from build123d import *

# Parameters (mm, degrees)
EXTRUDE_1_DEPTH = 46
SKETCH_2_R      = 5
EXTRUDE_2_DEPTH = 113
FILLET_1_R      = 3


with BuildPart() as part:
    # 草圖1 → 填料-伸長1 (new body)
    with BuildSketch(Plane.XY):
        Polygon((-15, 1.25), (-13.544119063, 5.25), (13.544119063, 5.25), (15, 1.25), (15, -1.25), (13.544119063, -5.25), (-13.544119063, -5.25), (-15, -1.25), align=None)
    extrude(amount=EXTRUDE_1_DEPTH)

    # 草圖2 → 填料-伸長2 (add)
    with BuildSketch(Plane(origin=(0, 0, 0), x_dir=(-1, 0, 0), z_dir=(0, 0, -1))):
        with Locations((7, 0)):
            Circle(SKETCH_2_R)
    extrude(amount=EXTRUDE_2_DEPTH)

    # 圓角1
    fillet_1_edges = [part.edges().sort_by_distance(p)[0] for p in [
        (-2, 0, -113),
    ]]
    fillet(fillet_1_edges, radius=FILLET_1_R)


solid = part.part
Verification items for the finished model (mm, model axes). A direction names the side the tool comes from. Coordinates: 2 decimals unless noted, no trailing zeros. Loops run counter-clockwise (first coordinate to the right, second up) from the corner with the lowest first, then second, coordinate; pieces in that order, holes last. Notation, with made-up numbers: (-36, 51) -> (-21, 51) arc R12 cw to (-21, 61) -> close; hole circle Ø9 at (-25.5, 4). An arc over 180 degrees is marked (long way). Answer as a JSON object with one key per item and string values. Group by question number.
Item 1: Tool access check on faces 1 (the flat face through (-7, 0, -113)), 2 (the cylindrical face through (-11.77, 1.5, -54.23)). Record the directions out of +Z, -Z, +X, -X, +Y, -Y that give a thin tool (end or side, any length) a straight path to the whole face; none if there is none.
Item 2: Sectioned sample at A-A on z = 5.5. Record the boundary of the cut face in (x, y), plus the area to 3 significant figures.
Item 3: Sectioned sample at C-C on z = -43. Record the boundary of the cut face in (x, y), plus the area to 3 significant figures.
Item 4: Scan lines: probe 1 along Z at (x, y) = (-1.75, -3); probe 2 along X at (y, z) = (-2.5, -13.5); probe 3 along X at (y, z) = (-4, -25). Record each from-to range of solid material in increasing order.
Item 5: Depth check by flat-ended pin: pin 1 (5 mm diameter, centred on x = -7, z = -17.5, fed in from -Y); pin 2 (1 mm diameter, centred on x = 0, z = -88, fed in from +Y) (3 decimals); pin 3 (3 mm diameter, centred on x = -11, y = 1, fed in from -Z); pin 4 (4 mm diameter, centred on x = -11, z = -69.5, fed in from +Y). Enter the tip coordinate at first touch or a pass-through.
Item 6: Sectioned sample at B-B on x = 5.25. Record the boundary of the cut face in (y, z), plus the area to 3 significant figures.
Evaluation:
{
 "1": {"face 1": "-Z, +X, -X, +Y, -Y", "face 2": "-Z"},
 "2": {"outline": "(-15, -1.25) -> (-13.54, -5.25) -> (13.54, -5.25) -> (15, -1.25) -> (15, 1.25) -> (13.54, 5.25) -> (-13.54, 5.25) -> (-15, 1.25) -> close", "area": "303 mm²"},
 "3": {"outline": "circle Ø10 at (-7, 0)", "area": "78.5 mm²"},
 "4": {"probe 1": "z = 0 to 46", "probe 2": "x = -11.33 to -2.67", "probe 3": "x = -10 to -4"},
 "5": {"pin 1": "stops at y = -5", "pin 2": "passes through", "pin 3": "stops at z = -112.93", "pin 4": "stops at y = 4.58"},
 "6": {"outline": "(-5.25, 0) -> (5.25, 0) -> (5.25, 46) -> (-5.25, 46) -> close", "area": "483 mm²"}
}
